Can you work these out from the model? Positions are in its coordinate system, mm. Face numbers are marked on the shaded views. A direction names the side the tool comes from. Give positions to 0.01 mm unless a question says otherwise; leave off trailing zeros. Write each loop counter-clockwise with the first axis right and the second up, starting at its lowest first coordinate (ties: lowest second). Pieces come first, ordered by that corner, then holes.
1. I'm going to push flat-ended pins straight in: pin 1 (3 mm diameter, centred on y = -8.5, z = -1.5, fed in from +X); pin 2 (7 mm diameter, centred on x = -29, y = -11, fed in from +Z); pin 3 (11.5 mm diameter, centred on x = -31.5, y = -15, fed in from -Z). Where does each tip first touch, or does it pass through?
2. Suppose I cut it at C-C (x = -1.5). Please give me the cut outline in (y, z).
3. On a 3-axis mill with a long thin cutter (end or side, diameter ignored), from which of +Z, -Z, +X, -X, +Y, -Y can I reach the whole of each face in a straight line? I mean the marked faces 1, 2 and 3. Say none if no direction works.
4. Thinking about a two-plate mould opening in X: for the marked faces 4, 5 and 6, which applies, pulls with the +X half, pulls with the -X half, needs draft (parallel to the pull), parting line crosses it, or undercut?
5. Suppose I cut it at B-B (x = 11). Please give me the cut outline in (y, z), and give its area (3 significant figures).
6. Suppose I cut it at D-D (z = 12.5). Please give me the cut outline in (x, y).
7. If I drill on probe 1 along Z at (x, y) = (-26.5, -2.5); probe 2 along Z at (x, y) = (13, -19); probe 3 along Z at (x, y) = (9.5, -2.25), over which ranges is the centre line in solid material (lowest first)?
8. Suppose I cut it at A-A (y = -8.5). Please give me the cut outline in (x, z), and give its area (3 significant figures).
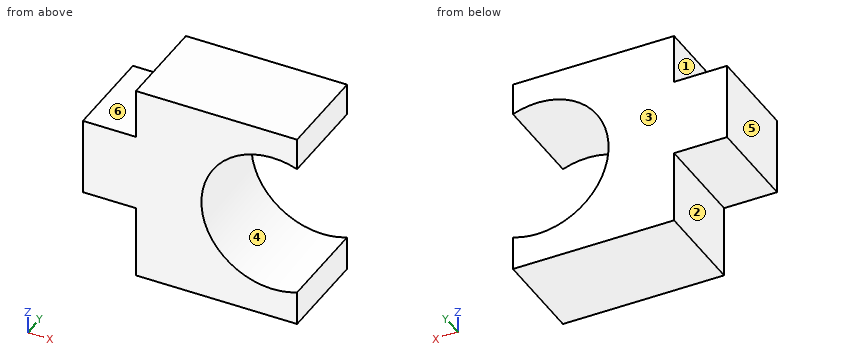
```python
from build123d import *

# Parameters (mm, degrees)
F1_DEPTH = 25.4


with BuildPart() as f1:
    # F0 (on Front) → F1 (new body)
    with BuildSketch(Plane.XZ):
        with BuildLine():
            Line((-23.929596, -11.450972), (-23.929596, -30.829543))
            Line((-23.929596, -30.829543), (18.938147, -30.829543))
            Line((18.938147, -30.829543), (18.938147, -21.727486))
            ThreePointArc((18.938147, -21.727486), (-6.506098, -3.963798), (18.938147, 13.79989))
            Line((18.938147, 13.79989), (18.938147, 22.314714))
            Line((18.938147, 22.314714), (-23.929596, 22.314714))
            Line((-23.929596, 22.314714), (-23.929596, 9.102055))
            Line((-23.929596, 9.102055), (-38.023103, 9.102055))
            Line((-38.023103, 9.102055), (-38.023103, -11.450972))
            Line((-38.023103, -11.450972), (-23.929596, -11.450972))
        make_face()
    extrude(amount=F1_DEPTH)


solid = f1.part
```
Checks:
1. pin 1: stops at x = -6.09
1. pin 2: stops at z = 9.1
1. pin 3: stops at z = -11.45
2. outline: (-25.4, -30.83) - (0, -30.83) - (0, -16.79) - (-25.4, -16.79) - close; (-25.4, 8.86) - (0, 8.86) - (0, 22.31) - (-25.4, 22.31) - close
3. face 1: +Z, -X, +Y, -Y
3. face 2: -Z, -X, +Y, -Y
3. face 3: +Z, -Z, +X, -X, +Y
4. face 4: undercut
4. face 5: pulls with the -X half
4. face 6: needs draft
5. outline: (-25.4, -30.83) - (0, -30.83) - (0, -22.83) - (-25.4, -22.83) - close; (-25.4, 14.91) - (0, 14.91) - (0, 22.31) - (-25.4, 22.31) - close
5. area: 391 mm2
6. outline: (-23.93, -25.4) - (3.09, -25.4) - (3.09, 0) - (-23.93, 0) - close
7. probe 1: z = -11.45 to 9.1
7. probe 2: z = -30.83 to -22.88, 14.95 to 22.31
7. probe 3: z = -30.83 to -22.66, 14.73 to 22.31
8. outline: (-38.02, -11.45) - (-23.93, -11.45) - (-23.93, -30.83) - (18.94, -30.83) - (18.94, -21.73) arc R18.92 cw (long way) to (18.94, 13.8) - (18.94, 22.31) - (-23.93, 22.31) - (-23.93, 9.1) - (-38.02, 9.1) - close
8. area: 1,760 mm2
